from build123d import *

# Parameters (mm, degrees)
SKETCH1_W           = 76.2
SKETCH1_H           = 63.5
BOSS_EXTRUDE1_DEPTH = 3.175
SKETCH2_W           = 15.875
SKETCH2_H           = 3.175
CUT_EXTRUDE1_DEPTH  = 50.6966108
CUT_EXTRUDE2_DEPTH  = 50.6966108


with BuildPart() as part:
    # Sketch1 → Boss-Extrude1 (new body)
    with BuildSketch(Plane.XY):
        Rectangle(SKETCH1_W, SKETCH1_H)
    extrude(amount=BOSS_EXTRUDE1_DEPTH)

    # Sketch2 → Cut-Extrude1 (cut, through all)
    with BuildSketch(Plane(origin=(0, 0, 0), x_dir=(-1, 0, 0), z_dir=(0, 0, -1))):
        with Locations((-30.1625, -30.1625)):
            Rectangle(SKETCH2_W, SKETCH2_H)
        with Locations((30.1625, -30.1625)):
            Rectangle(SKETCH2_W, SKETCH2_H)
        with Locations((30.1625, 30.1625)):
            Rectangle(SKETCH2_W, SKETCH2_H)
        with Locations((-30.1625, 30.1625)):
            Rectangle(SKETCH2_W, SKETCH2_H)
    extrude(amount=-CUT_EXTRUDE1_DEPTH, mode=Mode.SUBTRACT)

    # Sketch3 → Cut-Extrude2 (cut, through all)
    with BuildSketch(Plane.XY.offset(3.175)):
        Polygon((31.6625, -17.575), (31.6625, -20.125), (32.9625, -20.125), (32.9625, -22.025), (31.6625, -22.025), (31.6625, -28.575), (28.6625, -28.575), (28.6625, -22.025), (27.3625, -22.025), (27.3625, -20.125), (28.6625, -20.125), (28.6625, -17.575), align=None)
        Polygon((-31.6625, -20.125), (-32.9625, -20.125), (-32.9625, -22.025), (-31.6625, -22.025), (-31.6625, -28.575), (-28.6625, -28.575), (-28.6625, -22.025), (-27.3625, -22.025), (-27.3625, -20.125), (-28.6625, -20.125), (-28.6625, -17.575), (-31.6625, -17.575), align=None)
        Polygon((31.6625, 20.125), (32.9625, 20.125), (32.9625, 22.025), (31.6625, 22.025), (31.6625, 28.575), (28.6625, 28.575), (28.6625, 22.025), (27.3625, 22.025), (27.3625, 20.125), (28.6625, 20.125), (28.6625, 17.575), (31.6625, 17.575), align=None)
        Polygon((-31.6625, 17.575), (-31.6625, 20.125), (-32.9625, 20.125), (-32.9625, 22.025), (-31.6625, 22.025), (-31.6625, 28.575), (-28.6625, 28.575), (-28.6625, 22.025), (-27.3625, 22.025), (-27.3625, 20.125), (-28.6625, 20.125), (-28.6625, 17.575), align=None)
    extrude(amount=-CUT_EXTRUDE2_DEPTH, mode=Mode.SUBTRACT)


solid = part.part
Work out the finished part from the listing and answer in its coordinate system (mm). A direction names the side the tool comes from. Coordinates: 2 decimals unless noted, no trailing zeros. Write each loop counter-clockwise with the first axis right and the second up, starting at its lowest first coordinate (ties: lowest second). Pieces come first, ordered by that corner, then holes. Notation, with made-up numbers: (42, 66) - (53, 66) arc R29 ccw to (53, 89) - close; hole circle Ø1 at (-8.5, -28). An arc over 180 degrees is marked (long way). One line per question, with ' | ' between items.
1) For faces 1 (the face through (-31.662, 19, 2)), 2 (the face through (-28.662, -19, 2)), 3 (the face through (27.362, 21, 2)), 4 (the face through (25, 28.575, 2)), determine the directions among +Z, -Z, +X, -X, +Y, -Y from which every point of the face is accessible in a straight line to the end or side of a thin tool.
Checks:
face 1: +Z, -Z, +Y | face 2: +Z, -Z, -Y | face 3: +Z, -Z | face 4: +Z, -Z, +X, +Y
2) The mould has two halves that part along X. Classify faces 5 (the face through (-1, 0, 0)), 6 (the face through (-32.962, 21, 2)), 7 (the face through (38.1, 0, 2)), 8 (the face through (-22.225, 30, 2)): +X half, -X half, draft (parallel to the pull), parting line (faces both ways), or undercut.
Checks:
face 5: draft | face 6: undercut | face 7: +X half | face 8: -X half
3) Flat-ended cylindrical pins translate along their axes: P1, Ø1.4, axis at x = -27.5, z = 2, coming from the -Y side (3 decimals); P2, Ø1, axis at x = 28, z = 1, coming from the +Y side (3 decimals). Find the tip coordinate at first contact, or state that the pin passes through.
Checks:
P1: y = -28.575 | P2: y = 28.575
4) Find section A-A, the plane y = 25.5. Determine the outline of the cut face in (x, z) (1 decimal).
Checks:
outline: (-38.1, 0) - (-31.7, 0) - (-31.7, 3.2) - (-38.1, 3.2) - close; (-28.7, 0) - (28.7, 0) - (28.7, 3.2) - (-28.7, 3.2) - close; (31.7, 0) - (38.1, 0) - (38.1, 3.2) - (31.7, 3.2) - close
5) Consider probe 1 along X at (y, z) = (18.5, 2.1); probe 2 along Y at (x, z) = (-32, 2.85) (3 decimals); probe 3 along Y at (x, z) = (-27, 2.9) (3 decimals). Determine where each line is inside the solid, lowest interval first. Write a range as [from, to].
Checks:
probe 1: [-38.1, -31.66], [-28.66, 28.66], [31.66, 38.1] | probe 2: [-28.575, -22.025], [-20.125, 20.125], [22.025, 28.575] | probe 3: [-28.575, 28.575]
